Source: three-view drawing plus pictorial views. Frame: mm from the lowest corner of the part. Give positions to 0.01 mm unless a question says otherwise; leave off trailing zeros. Loops run counter-clockwise (first coordinate to the right, second up) from the corner with the lowest first, then second, coordinate; pieces in that order, holes last. Notation, with made-up numbers: (-1, -28) - (43, -28) arc R30 ccw to (43, -2) - close; hole circle Ø5 at (74, -24). An arc over 180 degrees is marked (long way). Answer as a JSON object with one key per item and string values. Group by question number.
(1) Section query A-A (y = 149.5). Return loops of the section in (x, z) (3 decimals), plus the area to 3 significant figures.
(2) Pin query (flat end, axial travel): P1, Ø1, axis at y = 151.5, z = 1, coming from the -X side; P2, Ø1.6, axis at x = 2.5, z = 2, coming from the -Y side; P3, Ø1.6, axis at x = 1.5, z = 2, coming from the +Y side. Return the tip coordinate at first contact, or that it passes through.
(3) Material intervals for L1, parallel to Y at x = 32.5, z = 0.8; L2, parallel to X at y = 42.5, z = 0.7, sorted ascending.
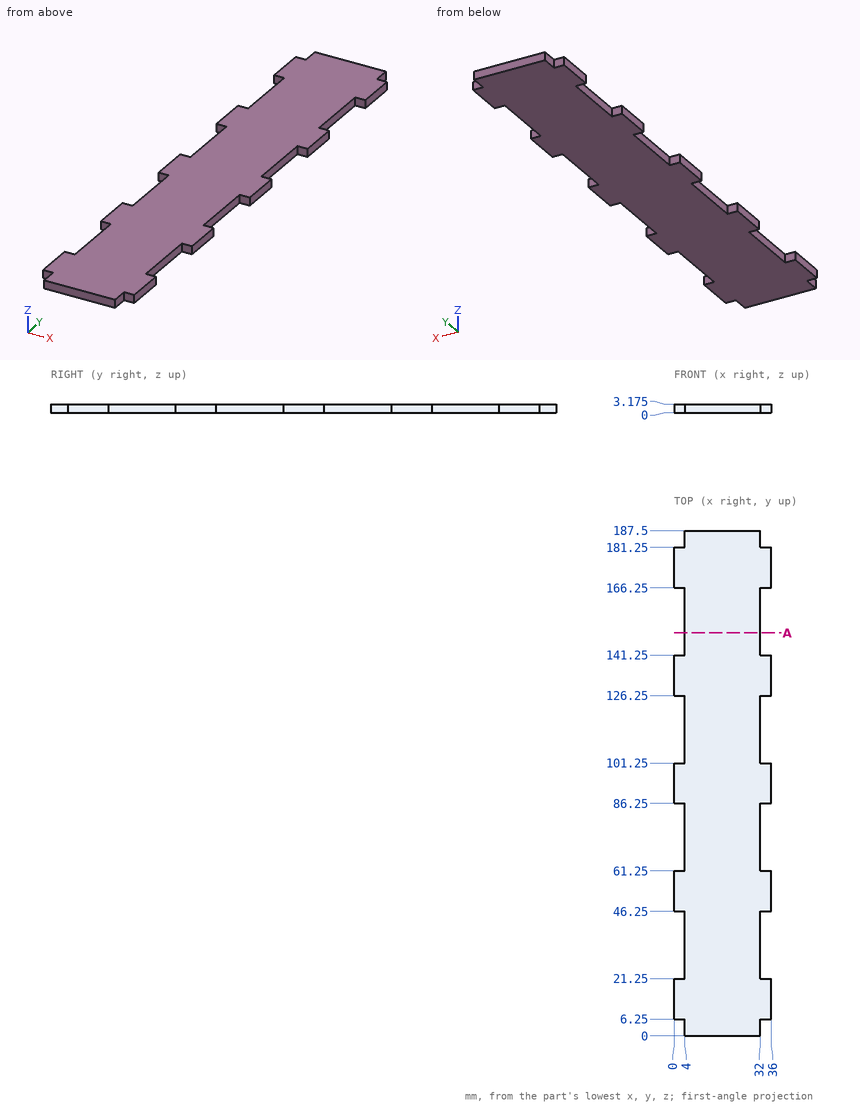
Recorded:
{
 "1": {"outline": "(4, 0) - (32, 0) - (32, 3.175) - (4, 3.175) - close", "area": "88.9 mm^2"},
 "2": {"P1": "stops at x = 4", "P2": "stops at y = 6.25", "P3": "stops at y = 181.25"},
 "3": {"L1": "y = 6.25 to 21.25, 46.25 to 61.25, 86.25 to 101.25, 126.25 to 141.25, 166.25 to 181.25", "L2": "x = 4 to 32"}
}
